Source: CAD feature listing. Evaluate the final solid. Frame: model axes, mm. Face numbers are marked on the shaded views. Round coordinates to 2 decimals unless told otherwise and drop trailing zeros. Loops run counter-clockwise (first coordinate to the right, second up) from the corner with the lowest first, then second, coordinate; pieces in that order, holes last. Notation, with made-up numbers: M -9.5,70 L 1.5,70 A33 ccw 1.5,109 Z; hole C 41,55.25 d1. An arc over 180 degrees is marked long. Answer as a JSON object with one key per item and string values.
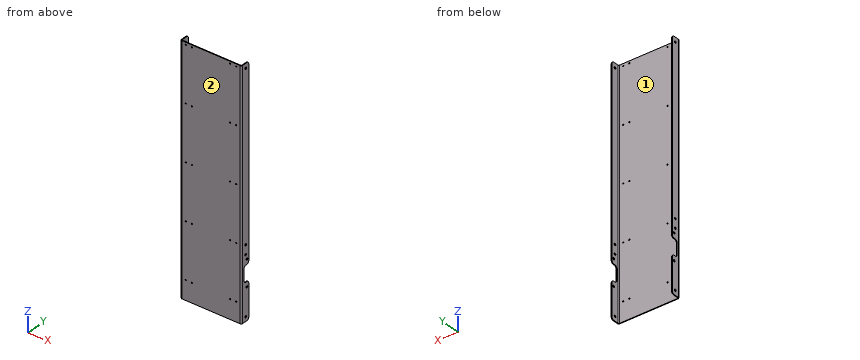
from build123d import *

# Parameters (mm, degrees)
SKETCH1_W                                 = 254
SKETCH1_H                                 = 1003.3
BASE_FLANGE1_DEPTH                        = 3.175
EDGE_FLANGE1_STRIP_W                      = 19.05
EDGE_FLANGE1_STRIP_H                      = 3.175
EDGE_FLANGE1_STRIP_CUT_DEPTH              = 1003.3
EDGE_FLANGE1_STRIP_2_W                    = 19.05
EDGE_FLANGE1_STRIP_2_H                    = 3.175
EDGE_FLANGE1_STRIP_CUT_2_DEPTH            = 1003.3
EDGE_FLANGE1_DEPTH                        = 1003.3
EDGE_FLANGE1_BEND_DEPTH                   = 1003.3
SKETCH30_W                                = 66.675
SKETCH30_H                                = 25.4
CUT_EXTRUDE4_DEPTH                        = 1036.541716024
HOLE_FOR_1_4_SELF_CLINCHING_NUTS_S_SS_C_D = 8.7376
F_10_0_1935_DIAMETER_HOLE1_D              = 4.9149
FILLET5_R                                 = 9.525


# Sheet-metal steps are written as plain solids
with BuildPart() as part:
    # Sketch1 → Base-Flange1 (new body)
    with BuildSketch(Plane(origin=(0, 0, 0), x_dir=(1, 0, 0), z_dir=(0, 1, 0))):
        with Locations((0, -501.65)):
            Rectangle(SKETCH1_W, SKETCH1_H)
    extrude(amount=-BASE_FLANGE1_DEPTH)

    # Edge-Flange1 strip (across the edge) → Edge-Flange1 strip cut (cut)
    with BuildSketch(Plane(origin=(-127, 0, 0), x_dir=(1, 0, 0), z_dir=(0, 0, 1))):
        with Locations((-3.175, -1.5875)):
            Rectangle(EDGE_FLANGE1_STRIP_W, EDGE_FLANGE1_STRIP_H)
    extrude(amount=EDGE_FLANGE1_STRIP_CUT_DEPTH, mode=Mode.SUBTRACT)

    # Edge-Flange1 strip 2 (across the edge) → Edge-Flange1 strip cut 2 (cut)
    with BuildSketch(Plane(origin=(127, 0, 1003.3), x_dir=(-1, 0, 0), z_dir=(0, 0, -1))):
        with Locations((-3.175, -1.5875)):
            Rectangle(EDGE_FLANGE1_STRIP_2_W, EDGE_FLANGE1_STRIP_2_H)
    extrude(amount=EDGE_FLANGE1_STRIP_CUT_2_DEPTH, mode=Mode.SUBTRACT)

    # Edge-Flange1 section (across the edge) → Edge-Flange1 (add)
    with BuildSketch(Plane(origin=(-127, 0, 0), x_dir=(1, 0, 0), z_dir=(0, 0, 1))):
        with BuildLine():
            Line((0, 3.175), (0, 34.925))
            Line((0, 34.925), (3.175, 34.925))
            Line((3.175, 34.925), (3.175, 3.175))
            ThreePointArc((3.175, 3.175), (4.10493597, 0.92993597), (6.35, 0))
            Line((6.35, 0), (6.35, -3.175))
            ThreePointArc((6.35, -3.175), (1.859871939, -1.315128061), (0, 3.175))
        make_face()
    extrude(amount=EDGE_FLANGE1_DEPTH)

    # Edge-Flange1 section 2 (across the edge) → Edge-Flange1 bend (add)
    with BuildSketch(Plane(origin=(127, 0, 1003.3), x_dir=(-1, 0, 0), z_dir=(0, 0, -1))):
        with BuildLine():
            Line((0, 3.175), (0, 34.925))
            Line((0, 34.925), (3.175, 34.925))
            Line((3.175, 34.925), (3.175, 3.175))
            ThreePointArc((3.175, 3.175), (4.10493597, 0.92993597), (6.35, 0))
            Line((6.35, 0), (6.35, -3.175))
            ThreePointArc((6.35, -3.175), (1.859871939, -1.315128061), (0, 3.175))
        make_face()
    extrude(amount=EDGE_FLANGE1_BEND_DEPTH)

    # Sketch30 → Cut-Extrude4 (cut, through all)
    with BuildSketch(Plane.ZY.offset(127)):
        with Locations((185.7375, 22.225)):
            Rectangle(SKETCH30_W, SKETCH30_H)
    extrude(amount=-CUT_EXTRUDE4_DEPTH, mode=Mode.SUBTRACT)

    # Hole for 1/4 Self-clinching Nuts (S,SS,CLS,CLSS)1 (through all)
    with Locations(Plane.ZY.offset(127)):
        with Locations((19.05, 19.05), (260.35, 19.05), (298.45, 19.05), (984.25, 19.05), (239.7125, 25.4), (131.7625, 25.4)):
            Hole(HOLE_FOR_1_4_SELF_CLINCHING_NUTS_S_SS_C_D / 2)

    # #10 (0.1935) Diameter Hole1 (through all)
    with Locations(Plane(origin=(0, 0, 0), x_dir=(1, 0, 0), z_dir=(0, 1, 0))):
        with Locations((104.775, -79.375), (79.375, -79.375), (-79.375, -79.375), (-104.775, -79.375), (-104.775, -307.975), (-79.375, -307.975), (79.375, -307.975), (104.775, -307.975), (104.775, -536.575), (79.375, -536.575), (-79.375, -765.175), (-79.375, -536.575), (-104.775, -536.575), (-104.775, -765.175), (79.375, -765.175), (104.775, -765.175), (104.775, -993.775), (79.375, -993.775), (-79.375, -993.775), (-104.775, -993.775)):
            Hole(F_10_0_1935_DIAMETER_HOLE1_D / 2)

    # Fillet5
    fillet5_edges = [part.edges().sort_by_distance(p)[0] for p in [
        (-125.4125, 34.925, 0),
        (-125.4125, 34.925, 1003.3),
        (125.4125, 34.925, 1003.3),
        (125.4125, 34.925, 0),
        (-125.4125, 34.925, 152.4),
        (-125.4125, 9.525, 219.075),
        (-125.4125, 9.525, 152.4),
        (-125.4125, 34.925, 219.075),
        (125.4125, 9.525, 152.4),
        (125.4125, 34.925, 152.4),
        (125.4125, 34.925, 219.075),
        (125.4125, 9.525, 219.075),
    ]]
    fillet(fillet5_edges, radius=FILLET5_R)


solid = part.part
Item 1: Section A-A on z = 940.5. Return the cut outline in (x, y) (3 decimals).
Answer sheet:
{"outline": "M -127,3.175 A6.35 ccw -120.65,-3.175 L 120.65,-3.175 A6.35 ccw 127,3.175 L 127,34.925 L 123.825,34.925 L 123.825,3.175 A3.175 cw 120.65,0 L -120.65,0 A3.175 cw -123.825,3.175 L -123.825,34.925 L -127,34.925 Z"}
Item 2: Pull-direction query (X, two-part tool) for the marked faces 1 and 2; classes: pulls with the +X half, pulls with the -X half, needs draft (parallel to the pull), parting line crosses it, or undercut.
Answer sheet:
{"face 1": "undercut", "face 2": "needs draft"}
Item 3: Section B-B on x = -31.5. Return the cut outline in (y, z) (3 decimals), then the cut area to 3 significant figures.
Answer sheet:
{"outline": "M -3.175,0 L 0,0 L 0,1003.3 L -3.175,1003.3 Z", "area": "3,190 mm²"}
Item 4: Line query: probe 1 along X at (y, z) = (14, 649) (3 decimals); probe 2 along Z at (x, y) = (125, 19); probe 3 along Y at (x, z) = (-10.5, 198) (3 decimals). Output: solid intervals per line, ascending. Write a range as from..to.
Answer sheet:
{"probe 1": "x = -127..-123.825, 123.825..127", "probe 2": "z = 0..14.68, 23.42..152.4, 219.07..255.98, 264.72..294.08, 302.82..979.88, 988.62..1003.3", "probe 3": "y = -3.175..0"}
Item 5: Contact query for a flat-ended pin moving along its axis: pin 1 Ø8 at (x, z) = (-104.775, 993.775) entering from +Y. Output: stop coordinate, or through.
Answer sheet:
{"pin 1": "stops at y = 0"}
